The figure shows three views and two pictorial views of one solid part (mm, origin at its lowest corner). Answer the questions. A direction names the side the tool comes from. Give positions to 0.01 mm unless a question says otherwise; leave off trailing zeros. Loops run counter-clockwise (first coordinate to the right, second up) from the corner with the lowest first, then second, coordinate; pieces in that order, holes last. Notation, with made-up numbers: (-2, 25) - (28, 25) arc R19 cw to (28, 40) - close; hole circle Ø2 at (19.25, -9). An arc over 180 degrees is marked (long way). Write item = value, one per line.
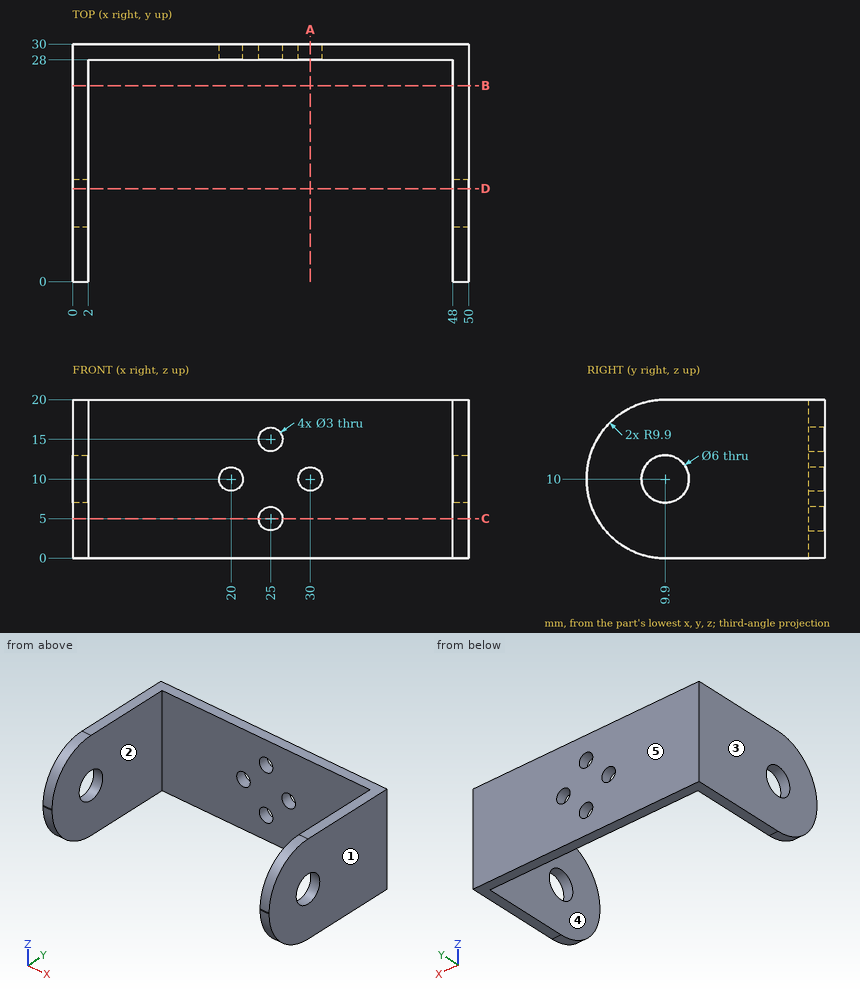
1) A cutting plane is placed at B-B on y = 24.75. Determine the outline of the cut face in (x, z).
Output:
outline = (0, 0) - (2, 0) - (2, 20) - (0, 20) - close; (48, 0) - (50, 0) - (50, 20) - (48, 20) - close
2) A cutting plane is placed at D-D on y = 11.75. Determine the outline of the cut face in (x, z), then the cut area to 3 significant figures.
Output:
outline = (0, 0) - (2, 0) - (2, 7.64) - (0, 7.64) - close; (0, 12.36) - (2, 12.36) - (2, 20) - (0, 20) - close; (48, 0) - (50, 0) - (50, 7.64) - (48, 7.64) - close; (48, 12.36) - (50, 12.36) - (50, 20) - (48, 20) - close
area = 61.1 mm²
3) Each of these flat-tipped pins is pushed along its axis until it touches: P1, Ø10, axis at x = 23, z = 11, coming from the -Y side; P2, Ø2.5, axis at x = 20, z = 10, coming from the +Y side. Where does it stop, or does it pass through?
Output:
P1 = 28
P2 = through
4) Find the intervals of material crossed by probe 1 along X at (y, z) = (28.8, 10); probe 2 along Y at (x, z) = (48.55, 10); probe 3 along X at (y, z) = (7, 13.5), in increasing order.
Output:
probe_1 = 0 to 18.5, 21.5 to 28.5, 31.5 to 50
probe_2 = 0 to 6.9, 12.9 to 30
probe_3 = 0 to 2, 48 to 50
5) A tool of negligible diameter and unlimited length cuts with its end or side. For the marked faces 4 and 5, from which of +Z, -Z, +X, -X, +Y, -Y can it reach the whole face along a straight path? Write none if from no direction.
Output:
face_4 = +Z, -Z, -Y
face_5 = +Z, -Z, +X, -X, +Y
6) The mould has two halves that part along X. Classify the marked faces 1, 2 and 3: pulls with the +X half, pulls with the -X half, needs draft (parallel to the pull), parting line crosses it, or undercut.
Output:
face_1 = pulls with the +X half
face_2 = undercut
face_3 = pulls with the -X half
7) A cutting plane is placed at C-C on z = 5. Determine the outline of the cut face in (x, y), then the cut area to 3 significant figures.
Output:
outline = (0, 1.3) - (2, 1.3) - (2, 28) - (23.5, 28) - (23.5, 30) - (0, 30) - close; (26.5, 28) - (48, 28) - (48, 1.3) - (50, 1.3) - (50, 30) - (26.5, 30) - close
area = 201 mm²
8) A cutting plane is placed at A-A on x = 30. Determine the outline of the cut face in (y, z), then the cut area to 3 significant figures.
Output:
outline = (28, 0) - (30, 0) - (30, 8.5) - (28, 8.5) - close; (28, 11.5) - (30, 11.5) - (30, 20) - (28, 20) - close
area = 34.0 mm²
